Read the model definition and answer for the solid it produces. Units are mm, in the model's axes. Coordinates: 2 decimals unless noted, no trailing zeros. Order: outer loops, then holes, each group sorted by start corner. A loop starts at its lowest first (then second) coordinate and runs counter-clockwise, first axis right, second up. Notation, with made-up numbers: (-11.5, 47.5) - (-6.5, 47.5) arc R31 ccw to (-6.5, 76.5) - close; hole circle Ø3 at (46, 76). An arc over 180 degrees is marked (long way). Answer as a JSON object with one key per item and string values. Group by question number.
from build123d import *

# Parameters (mm, degrees)
F2_SIZE2 = 1
F2_SIZE  = 0.5
F3_SIZE2 = 0.5
F3_SIZE  = 1
F4_R     = 1


with BuildPart() as f1:
    # F0 (on Top) → F1 (revolve)
    with BuildSketch(Plane.XY):
        Polygon((0, -7), (-17, -7.25), (-17, -10.25), (-8, -10.25), (-8, -11.75), (0, -11.75), align=None)
    revolve(axis=Axis((-8.5, 0, 0), (1, 0, 0)))

    # F2
    f2_edges = [f1.edges().sort_by_distance(p)[0] for p in [
        (-17, 10.25, 0),
    ]]
    chamfer(f2_edges, length=F2_SIZE, length2=F2_SIZE2)

    # F3
    f3_edges = [f1.edges().sort_by_distance(p)[0] for p in [
        (0, 7, 0),
    ]]
    chamfer(f3_edges, length=F3_SIZE, length2=F3_SIZE2)

    # F4
    f4_edges = [f1.edges().sort_by_distance(p)[0] for p in [
        (0, 11.75, 0),
    ]]
    fillet(f4_edges, radius=F4_R)


solid = f1.part
1. Straight lines are drawn through the part: L1, parallel to Y at x = -11.75, z = -7.25; L2, parallel to Y at x = -3.25, z = -3.25; L3, parallel to Y at x = -13.25, z = -6.5. For each, find the intervals that lie inside material, in ascending order.
2. A cutting plane is placed at B-B on x = -9.5. Write down the section's boundary in (y, z), and give its area (3 significant figures).
3. A cutting plane is placed at A-A on x = -15. Write down the section's boundary in (y, z), and give its area (3 significant figures).
4. For a pull along Z with two mould halves and no side action, classify faces 1 (the flat face through (-8, -4, -10)), 2 (the cylindrical face through (-11.944, 2.222, 10.006)), 3 (the conical face through (-9.11, 5.66, 4.34)) as pulls with the +Z half, pulls with the -Z half, needs draft (parallel to the pull), parting line crosses it, or undercut.
5. Given pin 1 (2 mm diameter, centred on x = -10.5, z = 9, fed in from +Y); pin 2 (1 mm diameter, centred on x = -12, z = -9.5, fed in from -Y); pin 3 (1.5 mm diameter, centred on x = -4.5, z = 5.5, fed in from +Y), each flat-ended and moving along its own axis, determine where each tip first touches the part or whether it passes through.
Derived:
{
 "1": {"L1": "y = -7.25 to 7.25", "L2": "y = -11.29 to -6.25, 6.25 to 11.29", "L3": "y = -7.93 to -3.08, 3.08 to 7.93"},
 "2": {"outline": "circle Ø20.5 at (0, 0); hole circle Ø14.28 at (0, 0)", "area": "170 mm2"},
 "3": {"outline": "circle Ø20.5 at (0, 0); hole circle Ø14.44 at (0, 0)", "area": "166 mm2"},
 "4": {"face 1": "needs draft", "face 2": "parting line crosses it", "face 3": "undercut"},
 "5": {"pin 1": "stops at y = 6.41", "pin 2": "stops at y = -4.91", "pin 3": "stops at y = 10.75"}
}
